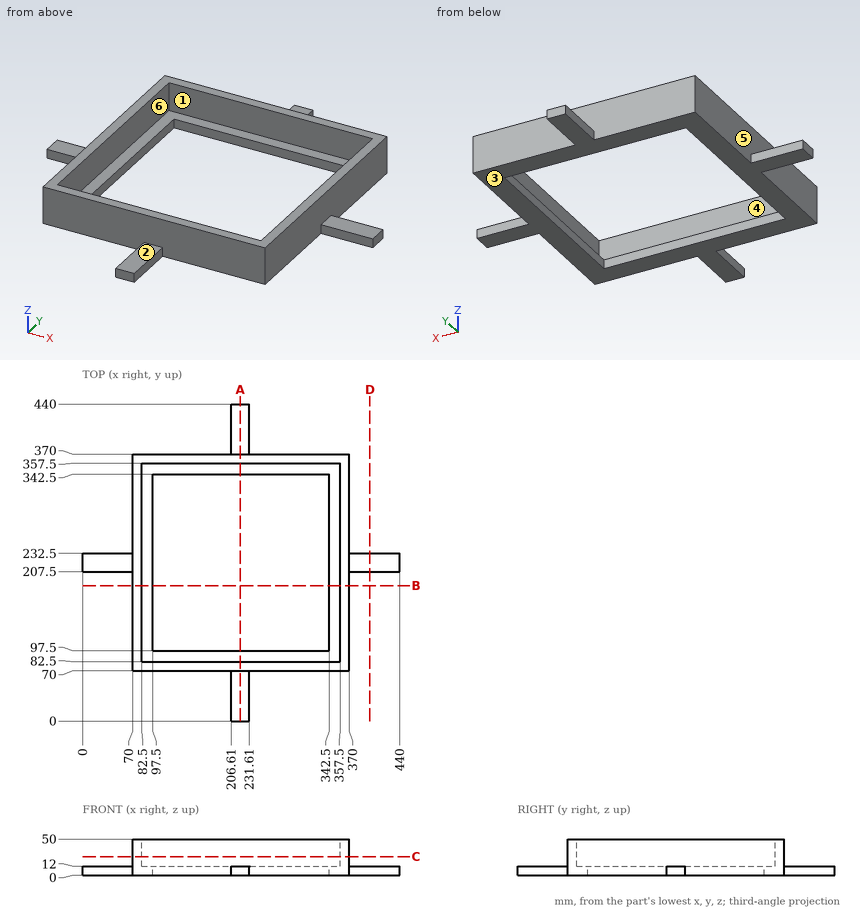
Here's the drawing with two shaded views (mm, measured from the low corner). I have some questions. A direction names the side the tool comes from. Coordinates: 2 decimals unless noted, no trailing zeros. Write each loop counter-clockwise with the first axis right and the second up, starting at its lowest first coordinate (ties: lowest second). Pieces come first, ordered by that corner, then holes. Notation, with made-up numbers: (37.25, 62.5) -> (85.25, 62.5) arc R36 ccw to (85.25, 98.5) -> close; hole circle Ø5 at (3, 22). An arc over 180 degrees is marked (long way). Use a Markdown table: item, result. Add a question column.
(1) If we section it at B-B, the plane y = 188: Write out the boundary of the cut face in (x, z), and give its area (3 significant figures).
(2) If we section it at D-D, the plane x = 399: Write out the boundary of the cut face in (y, z).
(3) I'm going to push flat-ended pins straight in: P1, Ø3, axis at y = 346, z = 7.5, coming from the +X side; P2, Ø6, axis at x = 97, y = 189.5, coming from the +Z side; P3, Ø19, axis at y = 215.5, z = 34, coming from the -X side. Where does each tip first touch, or does it pass through?
(4) For the marked faces 1, 2 and 3, which set-ups out of +Z, -Z, +X, -X, +Y, -Y let a thin tool reach every point of the face, with its end or its side?
(5) Please list where these lines run through material, in increasing order: line 1 (X direction, y = 156.5, z = 35); line 2 (X direction, y = 183.5, z = 5.5).
(6) We'd pull the mould along Y, two halves only. Please class the marked faces 4, 5 and 6: +Y half, -Y half, draft (parallel to the pull), parting line (faces both ways), or undercut.
(7) If we section it at A-A, the plane x = 219: Write out the boundary of the cut face in (y, z), and give its area (3 significant figures).
(8) If we section it at C-C, the plane z = 25.5: Write out the boundary of the cut face in (x, y), and give its area (3 significant figures).
Outcome:
| question | item | result |
|---|---|---|
| 1 | outline | (70, 0) -> (97.5, 0) -> (97.5, 12) -> (82.5, 12) -> (82.5, 50) -> (70, 50) -> close; (342.5, 0) -> (370, 0) -> (370, 50) -> (357.5, 50) -> (357.5, 12) -> (342.5, 12) -> close |
| 1 | area | 1,610 mm^2 |
| 2 | outline | (207.5, 0) -> (232.5, 0) -> (232.5, 12) -> (207.5, 12) -> close |
| 3 | P1 | stops at x = 370 |
| 3 | P2 | stops at z = 12 |
| 3 | P3 | stops at x = 70 |
| 4 | face 1 | +Z |
| 4 | face 2 | +Z, +X, -X, -Y |
| 4 | face 3 | -Z, +X, -X, +Y, -Y |
| 5 | line 1 | x = 70 to 82.5, 357.5 to 370 |
| 5 | line 2 | x = 70 to 97.5, 342.5 to 370 |
| 6 | face 4 | undercut |
| 6 | face 5 | draft |
| 6 | face 6 | undercut |
| 7 | outline | (0, 0) -> (97.5, 0) -> (97.5, 12) -> (82.5, 12) -> (82.5, 50) -> (70, 50) -> (70, 12) -> (0, 12) -> close; (342.5, 0) -> (440, 0) -> (440, 12) -> (370, 12) -> (370, 50) -> (357.5, 50) -> (357.5, 12) -> (342.5, 12) -> close |
| 7 | area | 3,290 mm^2 |
| 8 | outline | (70, 70) -> (370, 70) -> (370, 370) -> (70, 370) -> close; hole (82.5, 82.5) -> (357.5, 82.5) -> (357.5, 357.5) -> (82.5, 357.5) -> close |
| 8 | area | 14,400 mm^2 |
